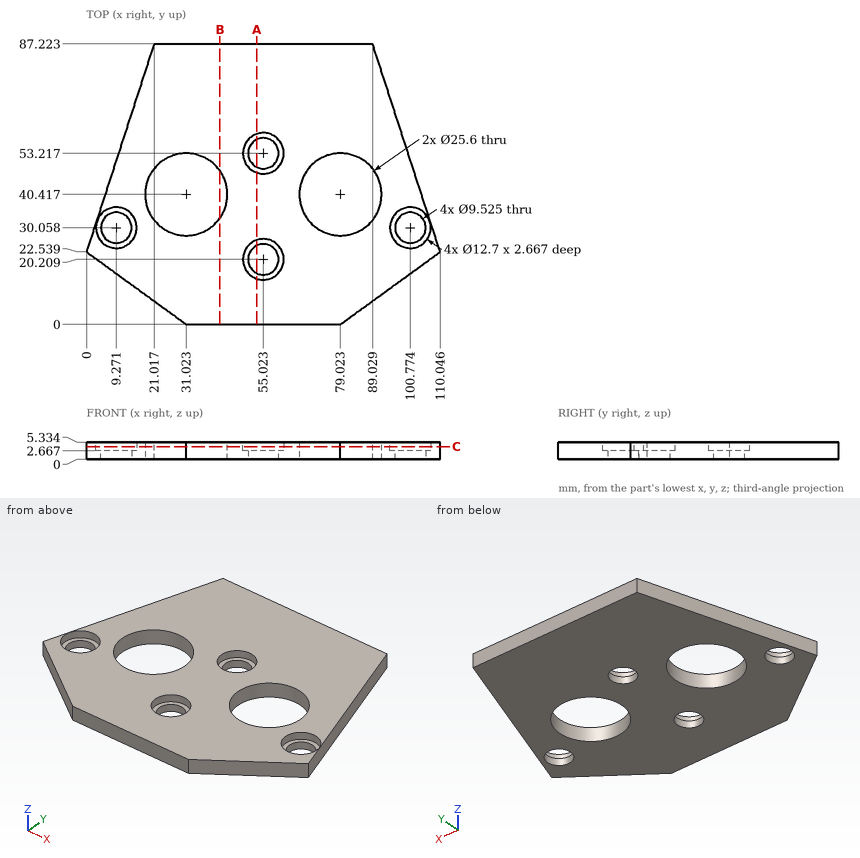
Geometry: see drawing. Coordinates: mm, zero at the bounding-box minimum. Round coordinates to 2 decimals unless told otherwise and drop trailing zeros. Loops run counter-clockwise (first coordinate to the right, second up) from the corner with the lowest first, then second, coordinate; pieces in that order, holes last.
(1) Section query C-C (z = 4). Give the number of separate pieces and of enclosed holes in the cut face, and give its area (3 significant figures).
From the geometry:
separate pieces: 1
enclosed holes: 6
area: 6,000 mm2
(2) Material intervals for probe 1 along X at (y, z) = (41, 3.1) (1 decimal); probe 2 along Y at (x, z) = (31, 1.6) (1 decimal); probe 3 along X at (y, z) = (32, 4.6) (1 decimal), sorted ascending.
From the geometry:
probe 1: x = 6 to 18.2, 43.8 to 66.2, 91.8 to 104
probe 2: y = 0 to 27.6, 53.2 to 87.2
probe 3: x = 3.1 to 3.2, 15.3 to 21.4, 40.7 to 69.4, 88.7 to 94.7, 106.8 to 107
(3) Contact query for flat-ended pins moving along their axis: pin 1 Ø5.5 at (x, y) = (9.27, 30.06) entering from +Z; pin 2 Ø11.5 at (x, y) = (100.77, 30.06) entering from +Z; pin 3 Ø2 at (y, z) = (29.5, 1.5) entering from -X; pin 4 Ø1.5 at (y, z) = (66.5, 4) entering from +X (1 decimal). Output: stop coordinate, or through.
From the geometry:
pin 1: passes through
pin 2: stops at z = 2.67
pin 3: stops at x = 1.94
pin 4: stops at x = 96
(4) Section query B-B (x = 41.5). Output: boundary loops of the cut face in (y, z) (1 decimal), and give its area (3 significant figures).
From the geometry:
outline: (0, 0) - (33.1, 0) - (33.1, 5.3) - (0, 5.3) - close; (47.8, 0) - (87.2, 0) - (87.2, 5.3) - (47.8, 5.3) - close
area: 387 mm2
(5) Section query A-A (x = 53). Output: boundary loops of the cut face in (y, z) (1 decimal), and give its area (3 significant figures).
From the geometry:
outline: (0, 0) - (15.9, 0) - (15.9, 2.7) - (14.2, 2.7) - (14.2, 5.3) - (0, 5.3) - close; (24.5, 0) - (48.9, 0) - (48.9, 2.7) - (47.2, 2.7) - (47.2, 5.3) - (26.2, 5.3) - (26.2, 2.7) - (24.5, 2.7) - close; (57.5, 0) - (87.2, 0) - (87.2, 5.3) - (59.2, 5.3) - (59.2, 2.7) - (57.5, 2.7) - close
area: 355 mm2
